Solid Edge part; units mm, degrees
sketch "Sketch1" plane through (0, 0, 0) normal (0, 0, 1) x (1, 0, 0)
  line L0 (23.075, -15.175) -> (23.075, 15.175)
  line L1 (23.075, 15.175) -> (-23.075, 15.175)
  line L2 (-23.075, 15.175) -> (-23.075, -15.175)
  line L3 (-23.075, -15.175) -> (23.075, -15.175)
extrude "Protrusion1" add sketch "Sketch1" against normal blind 3
sketch "Sketch2" plane through (0, 0, 0) normal (0, 0, 1) x (1, 0, 0)
  line L0 (-17.425, 13.9595) -> (-17.425, -14.0405)
  line L1 (-17.425, -14.0405) -> (12.075, -14.0405)
  line L2 (12.075, -14.0405) -> (12.075, 13.9595)
  line L3 (12.075, 13.9595) -> (-17.425, 13.9595)
extrude "ExtrudedProtrusion_2" add sketch "Sketch2" along normal blind 5.5
properties material "Glass, general industrial"
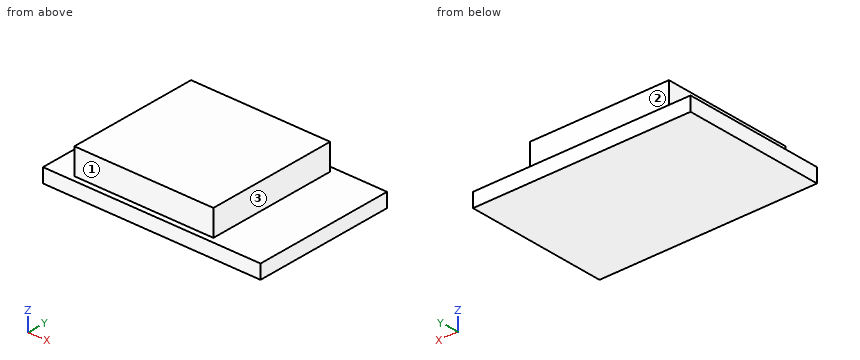
The listing builds one solid part. Answer for the finished solid, in the listing's coordinates (mm). Face numbers are marked on the shaded views. A direction names the side the tool comes from. Coordinates: 2 decimals unless noted, no trailing zeros. Order: outer loops, then holes, each group sorted by start corner. A loop starts at its lowest first (then second) coordinate and runs counter-clockwise, first axis right, second up. Notation, with made-up numbers: M 10.5,77 L 44.5,77 A37 cw 44.5,116 Z; hole C -11,-7 d4. An arc over 180 degrees is marked long. Use CSV: the item, a comma, the result in double quotes.
Q1. Straight lines are drawn through the part: L1, parallel to X at y = 11.5, z = 0.75 (3 decimals); L2, parallel to Y at x = 8, z = 5; L3, parallel to Z at x = -17.5, y = -12.5. For each, find the intervals that lie inside material, in ascending order.
Here are the results:
L1,"-17.425 to 12.075"
L2,"-14.04 to 13.96"
L3,"-3 to 0"
Q2. Section A-A (y = -6.5) is taken. Determine the outline of the cut face in (x, z) (3 decimals).
Here are the results:
outline,"M -23.075,-3 L 23.075,-3 L 23.075,0 L 12.075,0 L 12.075,5.5 L -17.425,5.5 L -17.425,0 L -23.075,0 Z"
Q3. A tool of negligible diameter and unlimited length cuts with its end or side. For the marked faces 1, 2 and 3, from which of +Z, -Z, +X, -X, +Y, -Y can it reach the whole face along a straight path? Write none if from no direction.
Here are the results:
face 1,"+Z, +X, -X, -Y"
face 2,"+Z, +X, -X, +Y"
face 3,"+Z, +X, +Y, -Y"
Q4. Section D-D (x = 14) is taken. Determine the outline of the cut face in (y, z) (3 decimals).
Here are the results:
outline,"M -15.175,-3 L 15.175,-3 L 15.175,0 L -15.175,0 Z"
Q5. Section B-B (x = 1) is taken. Determine the outline of the cut face in (y, z) (1 decimal).
Here are the results:
outline,"M -15.2,-3 L 15.2,-3 L 15.2,0 L 14,0 L 14,5.5 L -14,5.5 L -14,0 L -15.2,0 Z"
Q6. Section C-C (z = 2.25) is taken. Determine the outline of the cut face in (x, y) (1 decimal).
Here are the results:
outline,"M -17.4,-14 L 12.1,-14 L 12.1,14 L -17.4,14 Z"
Q7. Given pin 1 Ø2 at (y, z) = (11.5, 4) entering from +X (3 decimals); pin 2 Ø4.5 at (x, z) = (0, 2.5) entering from +Y; pin 3 Ø5 at (x, y) = (18, -6.5) entering from +Z, each flat-ended and moving along its own axis, determine where each tip first touches the part or whether it passes through.
Here are the results:
pin 1,"x = 12.075"
pin 2,"y = 13.96"
pin 3,"z = 0"
